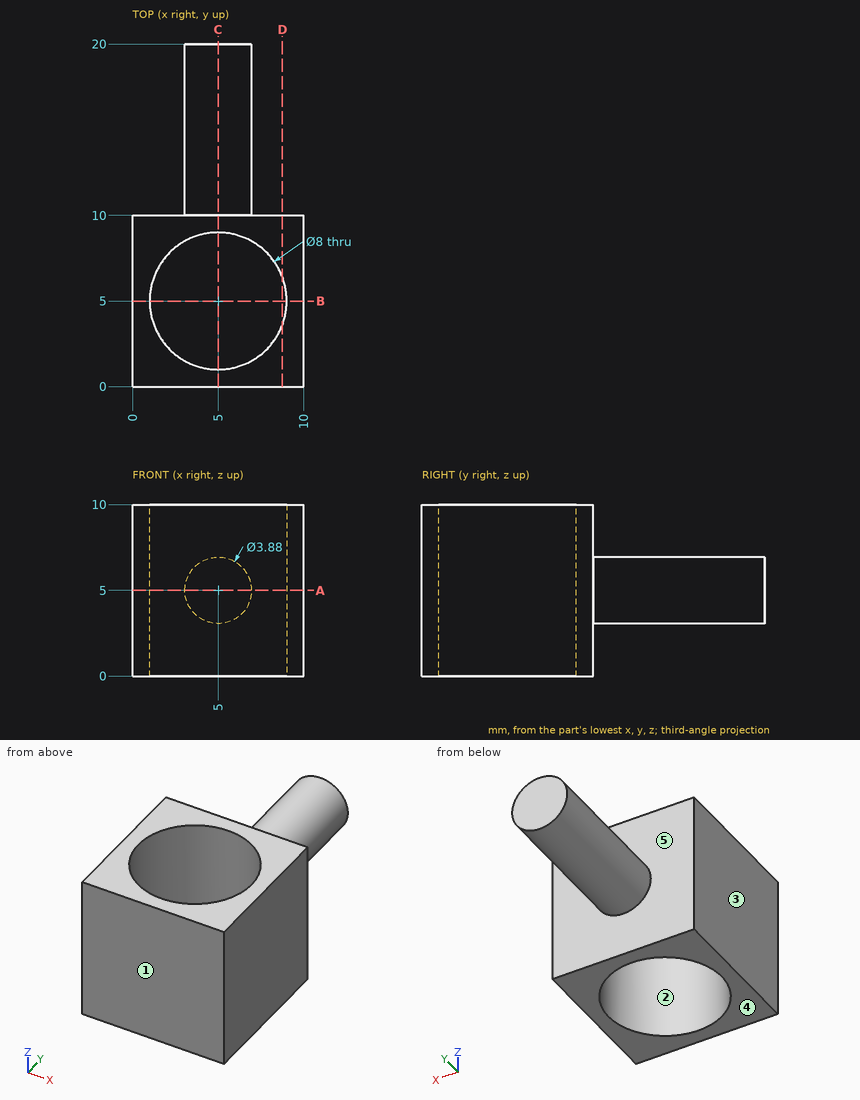
Could you check a few things on this drawing? It's one solid part, dimensions in mm from its lowest x, y, z. A direction names the side the tool comes from. Give positions to 0.01 mm unless a question says otherwise; leave off trailing zeros. Write each loop counter-clockwise with the first axis right and the second up, starting at its lowest first coordinate (ties: lowest second). Pieces come first, ordered by that corner, then holes. Notation, with made-up numbers: (54, 50) -> (71, 50) arc R19 ccw to (71, 85) -> close; hole circle Ø6 at (21.25, 31.5). An arc over 180 degrees is marked (long way). Write each question's results on one line, items separated by ' | '.
1. I want a section at A-A, the plane z = 5. Write out the boundary of the cut face in (x, y), then the cut area to 3 significant figures.
Check sheet entries:
outline: (0, 0) -> (10, 0) -> (10, 10) -> (6.94, 10) -> (6.94, 20) -> (3.06, 20) -> (3.06, 10) -> (0, 10) -> close; hole circle Ø8 at (5, 5) | area: 88.5 mm²
2. If we mould it in two halves opening along Y, with no side actions, what happens to the marked faces 1, 2 and 3? For each: released by +Y, released by -Y, zero draft, split by the parting line, or undercut.
Check sheet entries:
face 1: released by -Y | face 2: undercut | face 3: zero draft
3. On a 3-axis mill with a long thin cutter (end or side, diameter ignored), from which of +Z, -Z, +X, -X, +Y, -Y can I reach the whole of each face in a straight line? I mean the marked faces 4 and 5. Say none if no direction works.
Check sheet entries:
face 4: -Z, +X, -X, +Y, -Y | face 5: +Y
4. I need wall thicknesses on L1, parallel to Y at x = 5, z = 2.5; L2, parallel to X at y = 8.5, z = 3.5; L3, parallel to Y at x = 5, z = 5.75. Which ranges of each line are inside material? Lowest first, please.
Check sheet entries:
L1: y = 0 to 1, 9 to 10 | L2: x = 0 to 3.06, 6.94 to 10 | L3: y = 0 to 1, 9 to 20
5. I want a section at B-B, the plane y = 5. Write out the boundary of the cut face in (x, z).
Check sheet entries:
outline: (0, 0) -> (1, 0) -> (1, 10) -> (0, 10) -> close; (9, 0) -> (10, 0) -> (10, 10) -> (9, 10) -> close
6. I want a section at C-C, the plane x = 5. Write out the boundary of the cut face in (y, z), then the cut area to 3 significant figures.
Check sheet entries:
outline: (0, 0) -> (1, 0) -> (1, 10) -> (0, 10) -> close; (9, 0) -> (10, 0) -> (10, 3.06) -> (20, 3.06) -> (20, 6.94) -> (10, 6.94) -> (10, 10) -> (9, 10) -> close | area: 58.8 mm²
7. Will these pins go through, and if not, where does the flat tip stop? pin 1 Ø6 at (x, y) = (6.5, 18) entering from +Z; pin 2 Ø1.5 at (x, z) = (2, 5.5) entering from +Y; pin 3 Ø1.5 at (x, y) = (1, 11.5) entering from -Z.
Check sheet entries:
pin 1: stops at z = 6.94 | pin 2: stops at y = 10 | pin 3: passes through
8. I want a section at D-D, the plane x = 8.75. Write out the boundary of the cut face in (y, z), then the cut area to 3 significant figures.
Check sheet entries:
outline: (0, 0) -> (3.61, 0) -> (3.61, 10) -> (0, 10) -> close; (6.39, 0) -> (10, 0) -> (10, 10) -> (6.39, 10) -> close | area: 72.2 mm²
